Can you work these out from the model? Positions are in its coordinate system, mm. A direction names the side the tool comes from. Give positions to 0.01 mm unless a question says otherwise; leave off trailing zeros. Write each loop counter-clockwise with the first axis right and the second up, starting at its lowest first coordinate (ties: lowest second). Pieces come first, ordered by that corner, then holes. Notation, with made-up numbers: M -11,55.25 L 36,55.25 A29 ccw 36,83.25 Z; hole C 44,76.25 d8. An arc over 180 degrees is marked long. Write each question's results on one line, items separated by ' | '.
Autodesk Fusion 360 part; units mm, degrees
sketch "baseplate" plane through (0, 0, 0) normal (0, 1, 0) x (1, 0, 0)
  line L0 (0, 0) -> (80, 0)
  line L1 (80, 0) -> (80, -40)
  line L2 (80, -40) -> (0, -40)
  line L3 (0, -40) -> (0, 0)
  dimension "d1" = 40
  dimension "d2" = 80
extrude "Extrude1" add sketch "baseplate" along normal blind 10
sketch "outside_pryamid" plane through (0, 0, 0) normal (0, 1, 0) x (1, 0, 0)
  line L0 (5, -35) -> (15, -35)
  line L1 (15, -35) -> (15, -25)
  line L2 (15, -25) -> (5, -25)
  line L3 (5, -25) -> (5, -35)
  line L4 (25, -35) -> (35, -35)
  line L5 (35, -35) -> (35, -25)
  line L6 (35, -25) -> (25, -25)
  line L7 (25, -25) -> (25, -35)
  line L8 (45, -35) -> (55, -35)
  line L9 (55, -35) -> (55, -25)
  line L10 (55, -25) -> (45, -25)
  line L11 (45, -25) -> (45, -35)
  line L12 (65, -35) -> (75, -35)
  line L13 (75, -35) -> (75, -25)
  line L14 (75, -25) -> (65, -25)
  line L15 (65, -25) -> (65, -35)
  line L16 (25, -15) -> (35, -15)
  line L17 (35, -15) -> (35, -5)
  line L18 (35, -5) -> (25, -5)
  line L19 (25, -5) -> (25, -15)
  line L20 (5, -15) -> (15, -15)
  line L21 (15, -15) -> (15, -5)
  line L22 (15, -5) -> (5, -5)
  line L23 (5, -5) -> (5, -15)
  line L24 (45, -15) -> (55, -15)
  line L25 (55, -15) -> (55, -5)
  line L26 (55, -5) -> (45, -5)
  line L27 (45, -5) -> (45, -15)
  line L28 (65, -15) -> (75, -15)
  line L29 (75, -15) -> (75, -5)
  line L30 (75, -5) -> (65, -5)
  line L31 (65, -5) -> (65, -15)
  dimension "d5" = 10
  dimension "d6" = 10
ref_plane "WorkPlane1" through (0, 5, 0) normal (0, 1, 0) x (0, 0, 1)
sketch "inside_pryamid" plane through (0, 5, 0) normal (0, 1, 0) x (1, 0, 0)
  line L0 (47.5, -7.5) -> (47.5, -10)
  line L1 (47.5, -12.5) -> (52.5, -12.5)
  line L2 (52.5, -7.5) -> (47.5, -7.5)
  line L3 (47.5, -10) -> (47.5, -12.5)
  line L4 (52.5, -12.5) -> (52.5, -7.5)
  line L5 (67.5, -10) -> (67.5, -12.5)
  line L6 (67.5, -12.5) -> (72.5, -12.5)
  line L7 (67.5, -7.5) -> (67.5, -10)
  line L8 (72.5, -12.5) -> (72.5, -7.5)
  line L9 (72.5, -7.5) -> (67.5, -7.5)
  line L10 (67.5, -10) -> (67.5, -12.5)
  line L11 (67.5, -12.5) -> (72.5, -12.5)
  line L12 (72.5, -12.5) -> (72.5, -7.5)
  line L13 (47.5, -7.5) -> (47.5, -10)
  line L14 (52.5, -12.5) -> (52.5, -7.5)
  line L15 (72.5, -7.5) -> (67.5, -7.5)
  line L16 (47.5, -10) -> (47.5, -12.5)
  line L17 (52.5, -7.5) -> (47.5, -7.5)
  line L18 (67.5, -7.5) -> (67.5, -10)
  line L19 (47.5, -12.5) -> (52.5, -12.5)
  line L20 (72.5, -32.5) -> (72.5, -27.5)
  line L21 (72.5, -27.5) -> (67.5, -27.5)
  line L22 (67.5, -30) -> (67.5, -32.5)
  line L23 (72.5, -27.5) -> (67.5, -27.5)
  line L24 (67.5, -27.5) -> (67.5, -30)
  line L25 (47.5, -30) -> (47.5, -32.5)
  line L26 (67.5, -27.5) -> (67.5, -30)
  line L27 (67.5, -30) -> (67.5, -32.5)
  line L28 (67.5, -32.5) -> (72.5, -32.5)
  line L29 (72.5, -32.5) -> (72.5, -27.5)
  line L30 (47.5, -32.5) -> (52.5, -32.5)
  line L31 (47.5, -32.5) -> (52.5, -32.5)
  line L32 (67.5, -32.5) -> (72.5, -32.5)
  line L33 (52.5, -32.5) -> (52.5, -27.5)
  line L34 (52.5, -27.5) -> (47.5, -27.5)
  line L35 (52.5, -27.5) -> (47.5, -27.5)
  line L36 (47.5, -30) -> (47.5, -32.5)
  line L37 (52.5, -32.5) -> (52.5, -27.5)
  line L38 (47.5, -27.5) -> (47.5, -30)
  line L39 (47.5, -27.5) -> (47.5, -30)
loft "Loft3" cut profiles "outside_pryamid", "inside_pryamid" section 1 contours L8 L9 L10 L11 section 2 contours L25 L30 L31 L33 L34 L35 L36 L37 L38 L39
loft "Loft4" cut profiles "inside_pryamid", "outside_pryamid" section 1 contours L20 L21 L22 L23 L24 L26 L27 L28 L29 L32 section 2 contours L12 L13 L14 L15
loft "Loft7" cut profiles "inside_pryamid", "outside_pryamid" section 1 contours L0 L1 L2 L3 L4 L13 L14 L16 L17 L19 section 2 contours L24 L25 L26 L27
loft "Loft8" cut profiles "inside_pryamid", "outside_pryamid" section 1 contours L5 L6 L7 L8 L9 L10 L11 L12 L15 L18 section 2 contours L28 L29 L30 L31
sketch "sidewall" plane through (0, 0, 0) normal (0, 1, 0) x (1, 0, 0)
  line L0 (0, 0) -> (-8, 0)
  line L1 (-8, 0) -> (-8, -40)
  line L2 (-8, -40) -> (0, -40)
  line L3 (0, -40) -> (0, 0)
  dimension "d12" = 8
extrude "Extrude2" add sketch "sidewall" along normal blind -40 and the other way blind -10
sketch "sidemount" plane through (0, 0, 0) normal (0, 1, 0) x (1, 0, 0)
  line L0 (80, 0) -> (88, 0)
  line L1 (88, 0) -> (88, -40)
  line L2 (88, -40) -> (80, -40)
  line L3 (80, -40) -> (80, 0)
extrude "Extrude3" add sketch "sidemount" along normal blind 10
sketch "Sketch6" plane through (0, 0, 0) normal (0, 1, 0) x (1, 0, 0)
  circle A0 centre (-4, -34) radius 2
  circle A1 centre (-4, -6) radius 2
  circle A2 centre (-4, -34) radius 3.4
  circle A3 centre (-4, -6) radius 3.4
  line L0 (88, 0) -> (84, 0)
  line L1 (84, 0) -> (84, -6)
  line L2 (84, -6) -> (88, -6)
  line L3 (88, -6) -> (88, 0)
  circle A4 centre (84, -34) radius 2
  circle A5 centre (84, -6) radius 2
  dimension "d19" = 4
  dimension "d20" = 4
  dimension "d21" = 6.8
  dimension "d22" = 6.8
  dimension "d25" = 4
  dimension "d26" = 6
  dimension "d27" = 4
  dimension "d28" = 4
extrude "Extrude4" cut sketch "Sketch6" against normal blind 50 contours A0 | A1
extrude "Extrude5" cut sketch "Sketch6" along normal blind 40 contours L1 L2 A5 | L1 L2 A5 | A4
extrude "Extrude6" cut sketch "Sketch6" along normal through all and the other way blind 44 contours A0 | A1
extrude "Extrude7" cut sketch "Sketch6" along normal blind 10 and the other way blind -4 contours A2 | A3
sketch "45" plane through (0, 0, 0) normal (0, 0, 1) x (1, 0, 0)
  line L0 (45, 8) -> (40, 8)
  line L1 (40, 8) -> (40, 10)
  line L2 (40, 10) -> (40, 0)
  line L3 (40, 0) -> (0, -40)
  line L4 (0, -30) -> (47.3606, -30) construction
  line L5 (40, 0) -> (30, 0)
  line L6 (0, -30) -> (0, -40)
  line L7 (21.4627, -11.4663) -> (32.9289, 0)
  line L8 (21.4627, -11.4663) -> (-0.1828, -33.1117)
  line L9 (-0.1828, -33.1117) -> (0, 0)
  line L10 (0, 0) -> (32.9289, 0)
  dimension "d40" = 5
extrude "Extrude8" add sketch "45" along normal blind 40
sketch "Sketch8" plane through (0, 0, 40) normal (0, 0, 1) x (-1, 0, 0)
  line L0 (0, 40) -> (-40, 0)
  line L1 (-40, 0) -> (-88, 0)
  line L2 (-88, 0) -> (-88, -10)
  line L3 (-88, -10) -> (8, -10)
  line L4 (8, -10) -> (8, 40)
  line L5 (8, 40) -> (0, 40)
  line L6 (18.5559, 32.9289) -> (18.5559, -18.6929)
  line L7 (18.5559, -18.6929) -> (-38, -19)
  line L8 (-30, 0) -> (0, 30)
  line L9 (0, 30) -> (18.5559, 30)
  line L10 (-30, 0) -> (-46, -16)
  line L11 (-46, -16) -> (-38, -19)
extrude "Extrude10" cut sketch "Sketch8" against normal blind 50 contours L3 L4 L6 L7 L9 L10 L11 | L3 L4 L8 L9 L10
Item 1: I want a section at A-A, the plane x = 84. Please give me the cut outline in (y, z).
Geometry says:
outline: M 0,0 L 10,0 L 10,4 L 0,4 Z; M 0,8 L 10,8 L 10,32 L 0,32 Z; M 0,36 L 10,36 L 10,40 L 0,40 Z
Item 2: I want a section at B-B, the plane y = 7.5. Please give me the cut outline in (x, z).
Geometry says:
outline: M 37.5,0 L 88,0 L 88,40 L 37.5,40 Z; hole C 84,6 d4; hole C 84,34 d4
Item 3: I want a section at C-C, the plane z = 34. Give the number of separate pieces and of enclosed holes in the cut face, and give its area (3 significant figures).
Geometry says:
separate pieces: 3 | enclosed holes: 0 | area: 844 mm2
Item 4: Thinking about a two-plate mould opening in Z: for faces 1 (the face through (50, 5, 30)), 2 (the face through (33, -6, 0)), 3 (the face through (64, 0, 20)), which applies, +Z half, -Z half, draft (parallel to the pull), parting line (faces both ways), or undercut?
Geometry says:
face 1: undercut | face 2: -Z half | face 3: draft
Item 5: For faces 4 (the face through (-4, -30, 20)), 5 (the face through (85.908, 4.93, 6.601)), 6 (the face through (70, 5, 10)), which set-ups out of +Z, -Z, +X, -X, +Y, -Y let a thin tool reach every point of the face, with its end or its side?
Geometry says:
face 4: +Z, -Z, -X, +Y | face 5: +Y, -Y | face 6: -Y
Item 6: I'm going to push flat-ended pins straight in: pin 1 (1.5 mm diameter, centred on x = 51, z = 29.5, fed in from -Y); pin 2 (12 mm diameter, centred on x = 38, z = 22, fed in from -Y); pin 3 (4 mm diameter, centred on x = 69, z = 29, fed in from -Y); pin 4 (2.5 mm diameter, centred on x = -4, z = 34, fed in from -Y). Where does each tip first touch, or does it pass through?
Geometry says:
pin 1: stops at y = 5 | pin 2: stops at y = -8 | pin 3: stops at y = 4 | pin 4: passes through
Item 7: If I drill on line 1 (Z direction, x = -4, y = -36); line 2 (X direction, y = 5, z = 6); line 3 (X direction, y = -36, z = 34), over which ranges is the centre line in solid material (lowest first)? Write a range as from..to.
Geometry says:
line 1: z = 0..4, 8..32, 36..40 | line 2: x = 35..82, 86..88 | line 3: x = -8..-6, -2..4
